from build123d import *

# Parameters (mm, degrees)
SKETCH1_R               = 7.05
SKETCH1_W               = 6.5
SKETCH1_H               = 6.5
BOSS_EXTRUDE1_DEPTH     = 10
SKETCH2_R               = 17.5
BOSS_EXTRUDE2_DEPTH     = 6.5
CUT_EXTRUDE1_REACH      = 28.693
SKETCH3_R               = 1.25
CUT_EXTRUDE2_DEPTH      = 30.744747435
CUT_EXTRUDE2_DEPTH_BACK = 30.744747435
SKETCH4_R               = 1.5
CUT_EXTRUDE3_DEPTH      = 10
CUT_EXTRUDE3_DEPTH_BACK = 10
SKETCH6_W               = 6.5
SKETCH6_H               = 6.5
SKETCH8_W               = 5.75
SKETCH8_H               = 2.75
CUT_EXTRUDE4_DEPTH      = 5
CUT_EXTRUDE5_DEPTH      = 2.75
CIRPATTERN1_START       = 11.875
CIRPATTERN1_OUTLINE_R   = 1.25
CIRPATTERN1_DEPTH       = 2.75


# Read off the part's stored shape, not the designer's step: CirPattern1
with BuildPart() as part:
    # Sketch1 → Boss-Extrude1 (new body)
    with BuildSketch(Plane(origin=(0, 0, 0), x_dir=(1, 0, 0), z_dir=(0, 1, 0))):
        with Locations(Location((0, 0, 0), (0, 0, 270))):
            Circle(SKETCH1_R)
        Rectangle(SKETCH1_W, SKETCH1_H, mode=Mode.SUBTRACT)
    extrude(amount=BOSS_EXTRUDE1_DEPTH)

    # Sketch2 → Boss-Extrude2 (add)
    with BuildSketch(Plane(origin=(0, 10, 0), x_dir=(1, 0, 0), z_dir=(0, 1, 0))):
        with Locations(Location((0, 0, 0), (0, 0, 90))):
            Circle(SKETCH2_R)
    extrude(amount=BOSS_EXTRUDE2_DEPTH)

    # Sketch3 → Cut-Extrude1 (cut, up to next)
    with BuildSketch(Plane.XZ.offset(-10), mode=Mode.PRIVATE) as cut_extrude1_sk1:
        with Locations(Location((12.1, 0, 0), (0, 0, 270))):
            Circle(SKETCH3_R)
    cut_extrude1_tool1 = extrude(cut_extrude1_sk1.sketch, amount=-CUT_EXTRUDE1_REACH, mode=Mode.PRIVATE) & part.part
    # Sketch3 → Cut-Extrude1 (cut, up to next)
    with BuildSketch(Plane.XZ.offset(-10), mode=Mode.PRIVATE) as cut_extrude1_sk2:
        with Locations(Location((0, -12.1, 0), (0, 0, 270))):
            Circle(SKETCH3_R)
    cut_extrude1_tool2 = extrude(cut_extrude1_sk2.sketch, amount=-CUT_EXTRUDE1_REACH, mode=Mode.PRIVATE) & part.part
    # Sketch3 → Cut-Extrude1 (cut, up to next)
    with BuildSketch(Plane.XZ.offset(-10), mode=Mode.PRIVATE) as cut_extrude1_sk3:
        with Locations(Location((-12.1, 0, 0), (0, 0, 270))):
            Circle(SKETCH3_R)
    cut_extrude1_tool3 = extrude(cut_extrude1_sk3.sketch, amount=-CUT_EXTRUDE1_REACH, mode=Mode.PRIVATE) & part.part
    # Sketch3 → Cut-Extrude1 (cut, up to next)
    with BuildSketch(Plane.XZ.offset(-10), mode=Mode.PRIVATE) as cut_extrude1_sk4:
        with Locations(Location((0, 12.1, 0), (0, 0, 270))):
            Circle(SKETCH3_R)
    cut_extrude1_tool4 = extrude(cut_extrude1_sk4.sketch, amount=-CUT_EXTRUDE1_REACH, mode=Mode.PRIVATE) & part.part
    add(cut_extrude1_tool1.solids().sort_by_distance((12.1, 10, 0))[0], mode=Mode.SUBTRACT)
    add(cut_extrude1_tool2.solids().sort_by_distance((0, 10, -12.1))[0], mode=Mode.SUBTRACT)
    add(cut_extrude1_tool3.solids().sort_by_distance((-12.1, 10, 0))[0], mode=Mode.SUBTRACT)
    add(cut_extrude1_tool4.solids().sort_by_distance((0, 10, 12.1))[0], mode=Mode.SUBTRACT)

    # Sketch4 → Cut-Extrude2 (cut, two sides: drawn at the far end of the back side and taken through both)
    with BuildSketch(Plane.XY.offset(-CUT_EXTRUDE2_DEPTH_BACK)):
        with Locations((0, 4.916404418)):
            Circle(SKETCH4_R)
    extrude(amount=CUT_EXTRUDE2_DEPTH + CUT_EXTRUDE2_DEPTH_BACK, mode=Mode.SUBTRACT)

    # Sketch6 → Cut-Extrude3 (cut, two sides: drawn at the far end of the back side and taken through both)
    with BuildSketch(Plane(origin=(0, 10, 0), x_dir=(-1, 0, 0), z_dir=(0, -1, 0)).offset(-CUT_EXTRUDE3_DEPTH_BACK)):
        Rectangle(SKETCH6_W, SKETCH6_H)
    extrude(amount=CUT_EXTRUDE3_DEPTH + CUT_EXTRUDE3_DEPTH_BACK, mode=Mode.SUBTRACT)

    # Sketch8 → Cut-Extrude4 (cut)
    with BuildSketch(Plane(origin=(17.5, 0, 0), x_dir=(0, 0, -1), z_dir=(1, 0, 0))):
        with Locations((0, 13.25)):
            Rectangle(SKETCH8_W, SKETCH8_H)
    extrude(amount=-CUT_EXTRUDE4_DEPTH, mode=Mode.SUBTRACT)

    # Sketch9 → Cut-Extrude5 (cut)
    with BuildSketch(Plane.XZ.offset(-14.625)):
        Polygon((15.419764048, 0), (13.759882024, 2.875), (10.440117976, 2.875), (8.780235952, 0), (10.440117976, -2.875), (13.759882024, -2.875), align=None)
    extrude(amount=CUT_EXTRUDE5_DEPTH, mode=Mode.SUBTRACT)

    # CirPattern1 outline → CirPattern1 (cut)
    # profile 1 of 3: a face of its own
    with BuildSketch(Plane(origin=(0, 0, 0), x_dir=(1, 0, 0), z_dir=(0, 1, 0)).offset(CIRPATTERN1_START)):
        with BuildLine():
            Line((-8.780235952, 0), (-10.440117976, 2.875))
            Line((-10.440117976, 2.875), (-17.26222393, 2.875))
            ThreePointArc((-17.26222393, 2.875), (-17.5, 0), (-17.26222393, -2.875))
            Line((-17.26222393, -2.875), (-10.440117976, -2.875))
            Line((-10.440117976, -2.875), (-8.780235952, 0))
        make_face()
        with Locations((-12.1, 0)):
            Circle(CIRPATTERN1_OUTLINE_R, mode=Mode.SUBTRACT)
    # profile 2 of 3: a face of its own
    with BuildSketch(Plane(origin=(0, 0, 0), x_dir=(1, 0, 0), z_dir=(0, 1, 0)).offset(CIRPATTERN1_START)):
        with BuildLine():
            ThreePointArc((2.875, 17.26222393), (0, 17.5), (-2.875, 17.26222393))
            Line((-2.875, 17.26222393), (-2.875, 10.440117976))
            Line((-2.875, 10.440117976), (0, 8.780235952))
            Line((0, 8.780235952), (2.875, 10.440117976))
            Line((2.875, 10.440117976), (2.875, 17.26222393))
        make_face()
        with Locations((0, 12.1)):
            Circle(CIRPATTERN1_OUTLINE_R, mode=Mode.SUBTRACT)
    # profile 3 of 3: a face of its own
    with BuildSketch(Plane(origin=(0, 0, 0), x_dir=(1, 0, 0), z_dir=(0, 1, 0)).offset(CIRPATTERN1_START)):
        with BuildLine():
            Line((-2.875, -10.440117976), (-2.875, -17.26222393))
            ThreePointArc((-2.875, -17.26222393), (0, -17.5), (2.875, -17.26222393))
            Line((2.875, -17.26222393), (2.875, -10.440117976))
            Line((2.875, -10.440117976), (0, -8.780235952))
            Line((0, -8.780235952), (-2.875, -10.440117976))
        make_face()
        with Locations((0, -12.1)):
            Circle(CIRPATTERN1_OUTLINE_R, mode=Mode.SUBTRACT)
    extrude(amount=CIRPATTERN1_DEPTH, mode=Mode.SUBTRACT)


solid = part.part
Could you check a few things on this model? Use its own coordinates, in mm. A direction names the side the tool comes from. Coordinates: 2 decimals unless noted, no trailing zeros. Loops run counter-clockwise (first coordinate to the right, second up) from the corner with the lowest first, then second, coordinate; pieces in that order, holes last.
1. We'd pull the mould along Y, two halves only. Please class faces 1 (the face through (-0.195, 6.404, -5.178)), 2 (the face through (3.25, 8, 0)): released by +Y, released by -Y, zero draft, split by the parting line, or undercut.
2. For faces 3 (the face through (9.622, 13.269, 1.458)), 4 (the face through (-2.7, 4.93, 6.512)), 5 (the face through (-14, 11.875, 0)), 6 (the face through (-2.875, 13, 14)), which set-ups out of +Z, -Z, +X, -X, +Y, -Y let a thin tool reach every point of the face, with its end or its side?
3. Imagine slicing it at D-D (x = 10). Please give me the cut outline in (y, z) (3 decimals).
4. For P1, Ø6.5, axis at x = -0.5, z = 12.5, coming from the +Y side; P2, Ø3, axis at x = -1.5, y = 6.5, coming from the +Z side; P3, Ø1.4, axis at x = 14, y = 13, coming from the +Z side; P4, Ø3, axis at x = -13.5, z = 0.5, coming from the -Y side, each with a flat end and sliding along its axis, tell me the tip position at first contact or that it passes through.
5. I need wall thicknesses on L1, parallel to X at y = 10.75, z = 0; L2, parallel to X at y = 4.25, z = 0; L3, parallel to Y at x = 0, z = 6.25. Which ranges of each line are inside material? Lowest first, please.
6. Imagine slicing it at C-C (z = -14). Please give me the cut outline in (x, y) (3 decimals), and give its area (3 significant figures).
7. Imagine slicing it at A-A (y = 12.5). Please give me the cut outline in (x, z) (3 decimals), and give its area (3 significant figures).
8. Imagine slicing it at B-B (x = -12.1). Please give me the cut outline in (y, z) (3 decimals), and give its area (3 significant figures).
Computed values:
1. face 1: undercut
1. face 2: zero draft
2. face 3: +X
2. face 4: -Y
2. face 5: -X
2. face 6: +Z
3. outline: (10, -14.361) - (16.5, -14.361) - (16.5, 14.361) - (10, 14.361) - close; hole (11.875, -2.113) - (14.625, -2.113) - (14.625, 2.113) - (11.875, 2.113) - close
4. P1: stops at y = 16.5
4. P2: stops at z = 7.05
4. P3: stops at z = 11.37
4. P4: stops at y = 10
5. L1: x = -17.5 to -13.35, -10.85 to -3.25, 3.25 to 10.85, 13.35 to 17.5
5. L2: x = -7.05 to -3.25, 3.25 to 7.05
5. L3: y = 0 to 3.42, 6.42 to 16.5
6. outline: (-10.5, 10) - (10.5, 10) - (10.5, 16.5) - (-10.5, 16.5) - close; hole (-2.875, 11.875) - (2.875, 11.875) - (2.875, 14.625) - (-2.875, 14.625) - close
6. area: 121 mm2
7. outline: (-17.262, -2.875) arc R17.5 ccw to (-2.875, -17.262) - (-2.875, -10.44) - (0, -8.78) - (2.875, -10.44) - (2.875, -17.262) arc R17.5 ccw to (17.262, -2.875) - (10.44, -2.875) - (8.78, 0) - (10.44, 2.875) - (17.262, 2.875) arc R17.5 ccw to (2.875, 17.262) - (2.875, 10.44) - (0, 8.78) - (-2.875, 10.44) - (-2.875, 17.262) arc R17.5 ccw to (-17.262, 2.875) - (-10.44, 2.875) - (-8.78, 0) - (-10.44, -2.875) - close; hole (-3.25, -3.25) - (3.25, -3.25) - (3.25, 3.25) - (-3.25, 3.25) - close
7. area: 740 mm2
8. outline: (10, -12.643) - (16.5, -12.643) - (16.5, -1.25) - (14.625, -1.25) - (14.625, -2.875) - (11.875, -2.875) - (11.875, -1.25) - (10, -1.25) - close; (10, 1.25) - (11.875, 1.25) - (11.875, 2.875) - (14.625, 2.875) - (14.625, 1.25) - (16.5, 1.25) - (16.5, 12.643) - (10, 12.643) - close
8. area: 139 mm2
